Can you work these out from the model? Positions are in its coordinate system, mm. Face numbers are marked on the shaded views. A direction names the side the tool comes from. Coordinates: 2 decimals unless noted, no trailing zeros. Write each loop counter-clockwise with the first axis right and the second up, starting at its lowest first coordinate (ties: lowest second). Pieces come first, ordered by that corner, then holes. Notation, with made-up numbers: (66, -24.5) -> (102, -24.5) arc R14 cw to (102, -18.5) -> close; hole circle Ø11 at (55.5, 60). An arc over 180 degrees is marked (long way). Use one line per item in the form item = value.
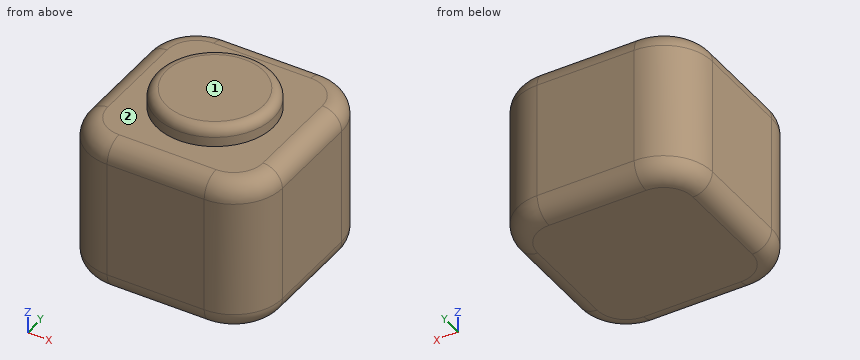
```python
from build123d import *

# Parameters (mm, degrees)
F0_W     = 12.7
F0_H     = 12.7
F1_DEPTH = 10.16
F2_R     = 3.175
F3_R     = 1.27
F4_R     = 3.81
F5_DEPTH = 1.27
F6_R     = 0.635
F7_R     = 1.27


with BuildPart() as f1:
    # F0 (on Top) → F1 (new body)
    with BuildSketch(Plane.XY):
        with Locations((6.35, 6.35)):
            Rectangle(F0_W, F0_H)
    extrude(amount=F1_DEPTH)

    # F2
    f2_edges = [f1.edges().sort_by_distance(p)[0] for p in [
        (0, 0, 5.08),
        (12.7, 0, 5.08),
        (12.7, 12.7, 5.08),
        (0, 12.7, 5.08),
    ]]
    fillet(f2_edges, radius=F2_R)

    # F3
    f3_edges = [f1.edges().sort_by_distance(p)[0] for p in [
        (6.35, 0, 10.16),
    ]]
    fillet(f3_edges, radius=F3_R)

    # F4 (on face) → F5 (join)
    with BuildSketch(Plane.XY.offset(10.16)):
        with Locations((6.35, 6.35)):
            Circle(F4_R)
    extrude(amount=F5_DEPTH)

    # F6
    f6_edges = [f1.edges().sort_by_distance(p)[0] for p in [
        (2.54, 6.35, 11.43),
    ]]
    fillet(f6_edges, radius=F6_R)

    # F7
    f7_edges = [f1.edges().sort_by_distance(p)[0] for p in [
        (0.929936, 0.929936, 0),
    ]]
    fillet(f7_edges, radius=F7_R)


solid = f1.part
```
Q1. If I drill on line 1 (Z direction, x = 9.75, y = 1.5); line 2 (Y direction, x = 6, z = 9), over which ranges is the centre line in solid material (lowest first)? Write a range as from..to.
Return value:
line_1 = 0..10.16
line_2 = 0..12.7
Q2. Suppose I cut it at A-A (z = 3.75). Write out the boundary of the cut face in (x, y) (3 decimals).
Return value:
outline = (0, 3.175) arc R3.175 ccw to (3.175, 0) -> (9.525, 0) arc R3.175 ccw to (12.7, 3.175) -> (12.7, 9.525) arc R3.175 ccw to (9.525, 12.7) -> (3.175, 12.7) arc R3.175 ccw to (0, 9.525) -> close
Q3. For the marked faces 1 and 2, which set-ups out of +Z, -Z, +X, -X, +Y, -Y let a thin tool reach every point of the face, with its end or its side?
Return value:
face_1 = +Z, +X, -X, +Y, -Y
face_2 = +Z
Q4. Suppose I cut it at B-B (x = 6.35). Write out the boundary of the cut face in (y, z) (3 decimals).
Return value:
outline = (0, 1.27) arc R1.27 ccw to (1.27, 0) -> (11.43, 0) arc R1.27 ccw to (12.7, 1.27) -> (12.7, 8.89) arc R1.27 ccw to (11.43, 10.16) -> (10.16, 10.16) -> (10.16, 10.795) arc R0.635 ccw to (9.525, 11.43) -> (3.175, 11.43) arc R0.635 ccw to (2.54, 10.795) -> (2.54, 10.16) -> (1.27, 10.16) arc R1.27 ccw to (0, 8.89) -> close
